Can you work these out from the drawing? Everything is in mm from the part's minimum corner. Round coordinates to 2 decimals unless told otherwise and drop trailing zeros. Loops run counter-clockwise (first coordinate to the right, second up) from the corner with the lowest first, then second, coordinate; pieces in that order, holes last. Notation, with made-up numbers: (83.5, -27.5) - (113.5, -27.5) arc R25 ccw to (113.5, 1.5) - close; hole circle Ø9 at (62, 11). An arc over 180 degrees is marked (long way). Answer as CSV lines item,"result". Start each with the question number.
1) Please list where these lines run through material, in increasing order: line 1 along Y through (x, z) = (15, 0.4) (1 decimal); line 2 along Y through (x, z) = (4.5, 0.25) (1 decimal); line 3 along Y through (x, z) = (13, 0.55) (1 decimal).
2) Suppose I cut it at B-B, the plane x = 5. Write out the boundary of the cut face in (y, z).
3) I'm going to push a flat-ended pin straight in: pin 1 Ø1.8 at (x, y) = (8.72, 15.11) entering from -Z. Where does the tip first touch, or does it pass through?
4) Suppose I cut it at A-A, the plane y = 5. Write out the boundary of the cut face in (x, z), then the cut area to 3 significant figures.
5) Suppose I cut it at C-C, the plane z = 0.8. Count the separate pieces of the cut face and the enclosed holes in it, then the cut area to 3 significant figures.
6) Suppose I cut it at D-D, the plane x = 9.5. Write out the boundary of the cut face in (y, z) (1 decimal).
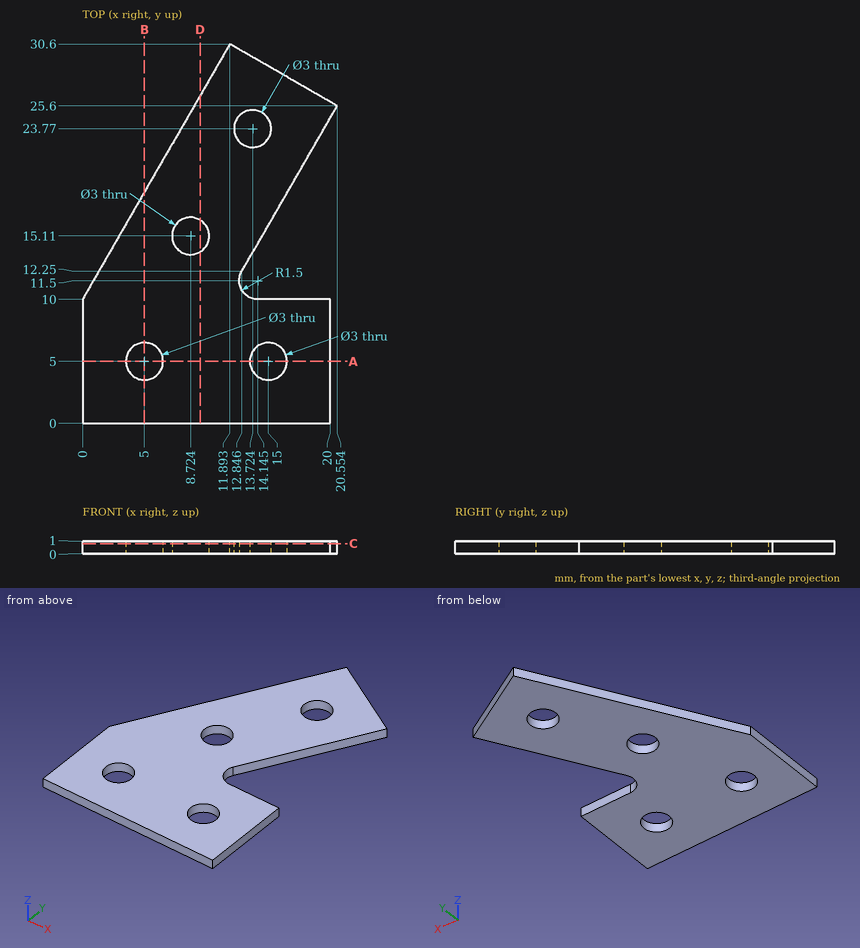
Filled sheet:
1,line 1,"0 to 3.5, 6.5 to 10, 16 to 23, 24.6 to 28.8"
1,line 2,"0 to 3.6, 6.4 to 17.8"
1,line 3,"0 to 10.5, 12.5 to 22.5, 25.1 to 30"
2,outline,"(0, 0) - (3.5, 0) - (3.5, 1) - (0, 1) - close; (6.5, 0) - (18.66, 0) - (18.66, 1) - (6.5, 1) - close"
3,pin 1,"through"
4,outline,"(0, 0) - (3.5, 0) - (3.5, 1) - (0, 1) - close; (6.5, 0) - (13.5, 0) - (13.5, 1) - (6.5, 1) - close; (16.5, 0) - (20, 0) - (20, 1) - (16.5, 1) - close"
4,area,"14.0 mm²"
5,separate pieces,"1"
5,enclosed holes,"4"
5,area,"382 mm²"
6,outline,"(0, 0) - (13.8, 0) - (13.8, 1) - (0, 1) - close; (16.4, 0) - (26.5, 0) - (26.5, 1) - (16.4, 1) - close"
